Can you work these out from the model? Positions are in its coordinate system, mm. Face numbers are marked on the shaded views. A direction names the side the tool comes from. Give positions to 0.01 mm unless a question says otherwise; leave off trailing zeros. Loops run counter-clockwise (first coordinate to the right, second up) from the corner with the lowest first, then second, coordinate; pieces in that order, holes last. Notation, with made-up numbers: (-8, -16.5) - (-1, -16.5) arc R9 cw to (-1, -7.5) - close; hole circle Ø4 at (28, -19.75). An arc over 180 degrees is marked (long way). Write item = value, one per line.
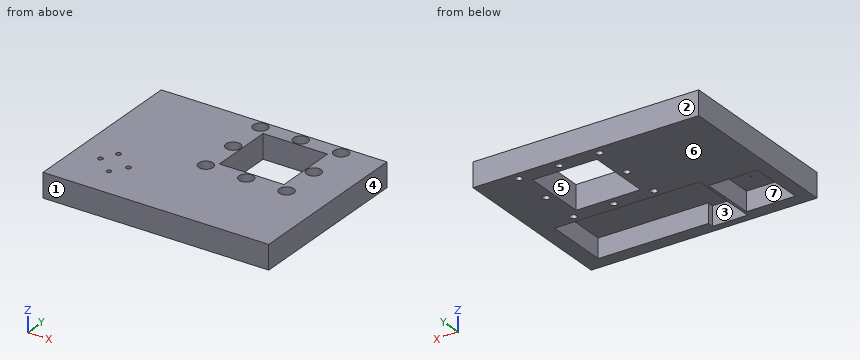
Autodesk Inventor part; units mm, degrees
ref_plane "Work Plane3" through (-75.6975, -60.1035, 12) normal (0, 0, 1) x (1, 0, 0)
ref_plane "YZ Plane" through (0, 0, 0) normal (1, 0, 0) x (0, 1, 0)
ref_plane "XZ Plane" through (0, 0, 0) normal (0, 1, 0) x (-1, 0, 0)
ref_plane "Work Plane1" through (0, 0, 0) normal (0, 0, 1) x (1, 0, 0)
ref_plane "Work Plane2" through (0, 0, 0) normal (0, 0, 1) x (1, 0, 0)
sketch "Sketch3" plane through (0, 0, 0) normal (0, 0, 1) x (1, 0, 0)
  circle A0 centre (0, 25) radius 1.95 construction
  circle A1 centre (-25, 0) radius 1.95 construction
  circle A2 centre (-25, -25) radius 1.95 construction
  circle A3 centre (25, 25) radius 1.95 construction
  circle A4 centre (25, -25) radius 1.95 construction
  circle A5 centre (-25, 25) radius 1.95 construction
  circle A6 centre (25, 0) radius 1.95 construction
  circle A7 centre (0, -25) radius 1.95 construction
  line L0 (-28, 30) -> (-30, 28) construction
  line L1 (-30, 28) -> (-30, -28) construction
  line L2 (-30, -28) -> (-28, -30) construction
  line L3 (-28, -30) -> (28, -30) construction
  line L4 (28, -30) -> (30, -28) construction
  line L5 (30, -28) -> (30, 28) construction
  line L6 (30, 28) -> (28, 30) construction
  line L7 (28, 30) -> (-28, 30) construction
  line L8 (30.0525, 30.0525) -> (-79.9475, 30.0525)
  line L9 (-79.9475, 30.0525) -> (-79.9475, -29.9475)
  line L10 (-79.9475, -29.9475) -> (30.0525, -29.9475)
  line L11 (30.0525, -29.9475) -> (30.0525, 30.0525)
  line L12 (-79.9475, -29.9475) -> (-49.9475, -29.9475)
  line L13 (-49.9475, -29.9475) -> (-49.9475, -69.9475)
  line L14 (-49.9475, -69.9475) -> (-79.9475, -69.9475)
  line L15 (-79.9475, -69.9475) -> (-79.9475, -29.9475)
  point P0 (0, 0)
  dimension "d5" = 110
  dimension "d6" = 60
  dimension "d7" = 30
  dimension "d8" = 40
extrude "Extrusion2" add sketch "Sketch3" along normal blind 12
sketch "Sketch4" plane through (0, 0, 12) normal (0, 0, 1) x (1, 0, 0)
  line L0 (-79.9475, 30.0525) -> (-79.9475, -69.9475)
  line L1 (-79.9475, -69.9475) -> (-49.9475, -69.9475)
  line L2 (-49.9475, -69.9475) -> (-49.9475, -29.9475)
  line L3 (-49.9475, -29.9475) -> (30.0525, -29.9475)
  line L4 (30.0525, -29.9475) -> (30.0525, 30.0525)
  line L5 (30.0525, 30.0525) -> (-79.9475, 30.0525)
  line L6 (-49.9475, -69.9475) -> (30.0525, -69.9475)
  line L7 (30.0525, -69.9475) -> (30.0525, -29.9475)
  line L8 (30.0525, -29.9475) -> (-49.9475, -29.9475)
  line L9 (-49.9475, -29.9475) -> (-49.9475, -69.9475)
  point P0 (0, 0)
extrude "Extrusion3" add sketch "Sketch4" along normal blind 3
sketch "Sketch5" plane through (0, 0, 15) normal (0, 0, 1) x (1, 0, 0)
  line L0 (-79.9475, -69.9475) -> (30.0525, -69.9475)
  line L1 (30.0525, -69.9475) -> (30.0525, 30.0525)
  line L2 (30.0525, 30.0525) -> (-79.9475, 30.0525)
  line L3 (-79.9475, 30.0525) -> (-79.9475, -69.9475)
  line L4 (-79.9475, -69.9475) -> (-49.9475, -69.9475)
  line L5 (-79.9475, -69.9475) -> (30.0525, -69.9475)
  line L6 (30.0525, -69.9475) -> (30.0525, -78.3535)
  line L7 (30.0525, -78.3535) -> (-79.9475, -78.3535)
  line L8 (-79.9475, -78.3535) -> (-79.9475, -69.9475)
  line L9 (30.0525, -78.3535) -> (34.0525, -78.3535)
  line L10 (34.0525, -78.3535) -> (34.0525, -24.0007)
  line L11 (34.0525, -24.0007) -> (30.0525, -24.0007)
  line L12 (30.0525, -24.0007) -> (30.0525, -78.3535)
  point P0 (0, 0)
  dimension "d13" = 110
  dimension "d14" = 8.406
  dimension "d15" = 4
  dimension "d16" = 54.353
extrude "Extrusion4" add sketch "Sketch5" against normal up to surface (15 mm away) contours L0 L6 L7 L8
sketch "Sketch6" plane through (0, 0, 15) normal (0, 0, 1) x (1, 0, 0)
  line L0 (30.0525, -78.3535) -> (30.0525, 30.0525)
  line L1 (30.0525, 30.0525) -> (-79.9475, 30.0525)
  line L2 (-79.9475, 30.0525) -> (-79.9475, -78.3535)
  line L3 (-79.9475, -78.3535) -> (30.0525, -78.3535)
  circle A0 centre (0, 25) radius 1.95
  circle A1 centre (-25, 0) radius 1.95
  circle A2 centre (-25, -25) radius 1.95
  circle A3 centre (25, 25) radius 1.95
  circle A4 centre (25, -25) radius 1.95
  circle A5 centre (-25, 25) radius 1.95
  circle A6 centre (25, 0) radius 1.95
  circle A7 centre (0, -25) radius 1.95
  line L4 (-28, 30) -> (-30, 28)
  line L5 (-30, 28) -> (-30, -28)
  line L6 (-30, -28) -> (-28, -30)
  line L7 (-28, -30) -> (28, -30)
  line L8 (28, -30) -> (30, -28)
  line L9 (30, -28) -> (30, 28)
  line L10 (30, 28) -> (28, 30)
  line L11 (28, 30) -> (-28, 30)
  point P0 (0, 0)
hole "Hole1" at (25, 25, 15) at (0, 25, 15) at (-25, 25, 15) at (-25, 0, 15) at (-25, -25, 15) at (0, -25, 15) at (25, -25, 15) at (25, 0, 15) direction (0, 0, -1) diameter 4.2 end through all counterbore diameter 9 counterbore depth 5
sketch "Sketch7" plane through (30.0525, -29.9475, 0) normal (1, 0, 0) x (0, 0, -1)
  line L0 (-10, 34.4475) -> (-10, 25.4475)
  line L1 (0, 0) -> (0, 60)
  line L2 (0, 60) -> (-15, 60)
  line L3 (-15, -48.406) -> (-15, 60)
  line L4 (-15, -48.406) -> (0, -48.406)
  line L5 (0, -48.406) -> (0, -40)
  line L6 (-12, -40) -> (0, -40)
  line L7 (-12, -40) -> (-12, 0)
  line L8 (0, 0) -> (-12, 0)
  point P0 (0, 29.9475)
extrude "Extrusion5" add sketch "Sketch7" along normal blind 10
sketch "Sketch8" plane through (40.0525, -29.9475, 0) normal (1, 0, 0) x (0, 0, -1)
  line L0 (0, 0) -> (0, 60)
  line L1 (0, 60) -> (-15, 60)
  line L2 (-15, 60) -> (-15, -48.406)
  line L3 (-15, -48.406) -> (0, -48.406)
  line L4 (0, -48.406) -> (0, -40)
  line L5 (0, -40) -> (-12, -40)
  line L6 (-12, -40) -> (-12, 0)
  line L7 (-12, 0) -> (0, 0)
  line L8 (0, 0) -> (-12, 0)
  line L9 (-12, 0) -> (-12, -40)
  line L10 (-12, -40) -> (0, -40)
  line L11 (0, -40) -> (0, 0)
  point P0 (0, 29.9475)
extrude "Extrusion6" add sketch "Sketch8" along normal blind 10
sketch "Sketch10" plane through (0, 0, 0) normal (0, 0, -1) x (-1, 0, 0)
  line L0 (49.9475, -29.9475) -> (-40.0525, -29.9475) construction
  line L1 (49.9475, -69.9475) -> (49.9475, -29.9475) construction
  line L2 (49.9475, -69.9475) -> (-40.0525, -69.9475) construction
  line L3 (-40.0525, -69.9475) -> (-40.0525, -29.9475) construction
  circle A0 centre (-25, -25) radius 2.1 construction
  circle A1 centre (25, -25) radius 2.1 construction
  circle A2 centre (25, 25) radius 2.1 construction
  circle A3 centre (-25, 25) radius 2.1 construction
  circle A4 centre (0, 25) radius 2.1 construction
  circle A5 centre (25, 0) radius 2.1 construction
  circle A6 centre (0, -25) radius 2.1 construction
  circle A7 centre (-25, 0) radius 2.1 construction
  line L4 (-50.0525, 30.0525) -> (79.9475, 30.0525) construction
  line L5 (-50.0525, -78.3535) -> (-50.0525, 30.0525) construction
  line L6 (79.9475, -78.3535) -> (-50.0525, -78.3535) construction
  line L7 (79.9475, 30.0525) -> (79.9475, -78.3535) construction
  line L8 (39, -67) -> (34, -67) construction
  line L9 (34, -71) -> (34, -67) construction
  line L10 (34, -71) -> (39, -71) construction
  line L11 (39, -67) -> (39, -71) construction
  line L12 (28.1949, -69.9475) -> (49.9475, -69.9475)
  line L13 (49.9475, -69.9475) -> (49.9475, -73.7985)
  line L14 (49.9475, -73.7985) -> (28.1949, -73.7985)
  line L15 (28.1949, -73.7985) -> (28.1949, -69.9475)
  point P0 (0, 0)
extrude "Extrusion8" cut sketch "Sketch10" against normal up to surface (12 mm away)
sketch "Sketch12" plane through (-79.9475, 30.0525, 0) normal (-1, 0, 0) x (0, 0, 1)
  line L0 (10, -97.0525) -> (10, -65.0525)
  line L1 (0, 0) -> (0, -108.406)
  line L2 (15, -108.406) -> (0, -108.406)
  line L3 (15, 0) -> (15, -108.406)
  line L4 (0, 0) -> (15, 0)
  point P0 (0, -30.0525)
extrude "Extrusion9" add sketch "Sketch12" along normal blind 10
sketch "Sketch15" plane through (0, 0, 0) normal (0, 0, -1) x (-1, 0, 0)
  circle A0 centre (0, 0) radius 7.5
  line L0 (20, -20) -> (-20, -20)
  line L1 (-20, -20) -> (-20, 20)
  line L2 (-20, 20) -> (20, 20)
  line L3 (20, 20) -> (20, -20)
  line L4 (20, -20) -> (-20, 20) construction
  line L5 (-20, -20) -> (20, 20) construction
  point P0 (0, 0)
  dimension "d52" = 40
  dimension "d53" = 40
extrude "Extrusion10" cut sketch "Sketch15" against normal through all contours A0 | L0 L1 L2 L3
sketch "Sketch16" plane through (0, 0, 0) normal (0, 0, -1) x (-1, 0, 0)
  circle A0 centre (65.0475, -49.3535) radius 8.5 construction
  line L0 (79.9475, -68.3535) -> (79.9475, -37.8535) construction
  line L1 (79.9475, -37.8535) -> (53.5475, -37.8535) construction
  line L2 (53.5475, -37.8535) -> (53.5475, -68.3535) construction
  line L3 (53.5475, -68.3535) -> (79.9475, -68.3535) construction
  line L4 (51.5475, -35.8535) -> (81.9475, -35.8535)
  line L5 (81.9475, -35.8535) -> (81.9475, -70.3535)
  line L6 (81.9475, -70.3535) -> (51.5475, -70.3535)
  line L7 (51.5475, -70.3535) -> (51.5475, -35.8535)
  point P0 (0, 0)
  dimension "d56" = 2
ref_plane "Work Plane3" through (-75.6975, -60.1035, 12) normal (0, 0, 1) x (1, 0, 0)
extrude "Extrusion11" cut sketch "Sketch16" against normal up to surface (12 mm away)
sketch "Sketch17" plane through (0, 0, 15) normal (0, 0, 1) x (1, 0, 0)
  circle A0 centre (-56.5475, -49.3535) radius 0.9
  circle A1 centre (-69.0475, -40.0535) radius 0.9
  arc A2 (-73.0475, -47.8527) -> (-73.0475, -50.8543) centre (-73.9475, -49.3535) ccw
  circle A3 centre (-62.5475, -58.3535) radius 0.9
  point P0 (0, 0)
hole "Hole4" at (-73.9475, -49.3535, 15) at (-69.0475, -40.0535, 15) at (-56.5475, -49.3535, 15) at (-62.5475, -58.3535, 15) direction (0, 0, -1) diameter 1 depth 10 tip angle 118 counterbore diameter 3 counterbore depth 2
properties part number "10_Baseplate_Axiotech_mono_zstagfe"
Q1. Imagine slicing it at B-B, the plane x = 0. Write out the boundary of the cut face in (y, z).
Output:
outline = (-78.35, 0) - (-69.95, 0) - (-69.95, 12) - (-29.95, 12) - (-29.95, 0) - (-27.1, 0) - (-27.1, 10) - (-29.5, 10) - (-29.5, 15) - (-78.35, 15) - close; (-22.9, 0) - (-20, 0) - (-20, 15) - (-20.5, 15) - (-20.5, 10) - (-22.9, 10) - close; (20, 0) - (22.9, 0) - (22.9, 10) - (20.5, 10) - (20.5, 15) - (20, 15) - close; (27.1, 0) - (30.05, 0) - (30.05, 15) - (29.5, 15) - (29.5, 10) - (27.1, 10) - close
Q2. We'd pull the mould along Y, two halves only. Please class the marked faces 1, 2, 3 and 4: released by +Y, released by -Y, zero draft, split by the parting line, or undercut.
Output:
face_1 = released by -Y
face_2 = released by +Y
face_3 = undercut
face_4 = zero draft
Q3. Which directions (+Z, -Z, +X, -X, +Y, -Y) give clear straight access to the entire face, cutting with the end or side of a thin tool? Please do the marked faces 5, 6 and 7.
Output:
face_5 = +Z, -Z
face_6 = -Z, +X, -X, +Y, -Y
face_7 = -Z
Q4. Imagine slicing it at D-D, the plane y = -53. Write out the boundary of the cut face in (x, z).
Output:
outline = (-89.95, 0) - (-81.95, 0) - (-81.95, 12) - (-51.55, 12) - (-51.55, 0) - (-49.95, 0) - (-49.95, 12) - (40.05, 12) - (40.05, 0) - (50.05, 0) - (50.05, 15) - (-89.95, 15) - close
Q5. Imagine slicing it at C-C, the plane z = 5.25. Give the number of separate pieces and of enclosed holes in the cut face, then the cut area to 3 significant figures.
Output:
separate_pieces = 1
enclosed_holes = 11
area = 8,730 mm2
Q6. I need wall thicknesses on L1, parallel to Y at x = 0, z = 3.5; L2, parallel to Y at x = -5, z = 11.25; L3, parallel to X at y = -37, z = 7.5. Which ranges of each line are inside material? Lowest first, please.
Output:
L1 = -78.35 to -69.95, -29.95 to -27.1, -22.9 to -20, 20 to 22.9, 27.1 to 30.05
L2 = -78.35 to -69.95, -29.95 to -20, 20 to 30.05
L3 = -89.95 to -81.95, -51.55 to -49.95, 40.05 to 50.05
Q7. Imagine slicing it at A-A, the plane y = -25. Write out the boundary of the cut face in (x, z), then the cut area to 3 significant figures.
Output:
outline = (-89.95, 0) - (-27.1, 0) - (-27.1, 10) - (-29.5, 10) - (-29.5, 15) - (-89.95, 15) - close; (-22.9, 0) - (-2.1, 0) - (-2.1, 10) - (-4.5, 10) - (-4.5, 15) - (-20.5, 15) - (-20.5, 10) - (-22.9, 10) - close; (2.1, 0) - (22.9, 0) - (22.9, 10) - (20.5, 10) - (20.5, 15) - (4.5, 15) - (4.5, 10) - (2.1, 10) - close; (27.1, 0) - (50.05, 0) - (50.05, 15) - (29.5, 15) - (29.5, 10) - (27.1, 10) - close
area = 1,840 mm2
Q8. For pin 1 (6.5 mm diameter, centred on x = 25, y = 25, fed in from -Z); pin 2 (4 mm diameter, centred on x = -25, y = 0, fed in from -Z); pin 3 (7 mm diameter, centred on x = 25, y = -25, fed in from +Z), each with a flat end and sliding along its axis, tell me the tip position at first contact or that it passes through.
Output:
pin_1 = 0
pin_2 = through
pin_3 = 10
